Work out the finished part from the listing and answer in its coordinate system (mm). Give positions to 0.01 mm unless a question says otherwise; leave off trailing zeros. Loops run counter-clockwise (first coordinate to the right, second up) from the corner with the lowest first, then second, coordinate; pieces in that order, holes last. Notation, with made-up numbers: (56, 6) -> (107, 6) arc R12 ccw to (107, 12) -> close; hole circle Ø9 at (78, 62). An arc over 180 degrees is marked (long way). Answer as CSV lines item,"result". Start each with the question number.
1. Flat-ended cylindrical pins translate along their axes: pin 1 Ø1 at (y, z) = (-6.5, 5.5) entering from -X; pin 2 Ø1 at (y, z) = (1.5, 35.5) entering from +X; pin 3 Ø2 at (y, z) = (-3.5, 24) entering from +X. Find the tip coordinate at first contact, or state that the pin passes through.
2. Find the intervals of material crossed by line 1 along Y through (x, z) = (0, 24.5); line 2 along X through (y, z) = (-7, 38); line 3 along X through (y, z) = (-7.75, 11.5), in increasing order.
3. Find section A-A, the plane x = -5.75. Give the vertices of the cut face in (y, z).
4. Find section B-B, the plane z = 12.5. Give the vertices of the cut face in (x, y).
5. Find section C-C, the plane y = -6.25. Give the vertices of the cut face in (x, z).
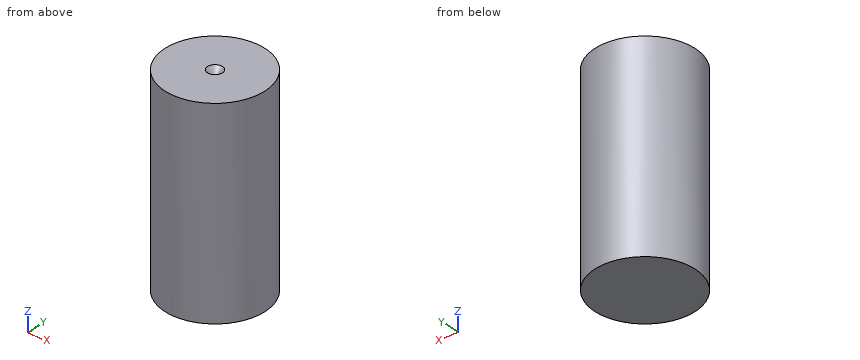
from build123d import *

# Parameters (mm, degrees)
F0_R     = 10
F1_DEPTH = 40
F2_R     = 1.5
F3_DEPTH = 1.5
F4_SIZE  = 1.49999


# Not quite as in the source:
# - a fillet or chamfer is up to 0.001 mm smaller than in the source, because OpenCascade refuses the exact size


with BuildPart() as f1:
    # F0 (on Top) → F1 (new body)
    with BuildSketch(Plane.XY):
        Circle(F0_R)
    extrude(amount=F1_DEPTH)

    # F2 (on face) → F3 (cut)
    with BuildSketch(Plane.XY.offset(40)):
        Circle(F2_R)
    extrude(amount=-F3_DEPTH, mode=Mode.SUBTRACT)

    # F4 (size 1.5 in the source; OpenCascade refuses exactly that, so slightly less here)
    f4_edges = [f1.edges().sort_by_distance(p)[0] for p in [
        (-1.5, 0, 38.5),
    ]]
    chamfer(f4_edges, length=F4_SIZE)


solid = f1.part
Resolved:
1,pin 1,"stops at x = -8"
1,pin 2,"stops at x = 9.95"
1,pin 3,"stops at x = 9.68"
2,line 1,"y = -10 to 10"
2,line 2,"x = -7.14 to 7.14"
2,line 3,"x = -6.32 to 6.32"
3,outline,"(-8.18, 0) -> (8.18, 0) -> (8.18, 40) -> (-8.18, 40) -> close"
4,outline,"circle Ø20 at (0, 0)"
5,outline,"(-7.81, 0) -> (7.81, 0) -> (7.81, 40) -> (-7.81, 40) -> close"
